```python
from build123d import *

# Parameters (mm, degrees)
BOSS_EXTRUDE1_DEPTH = 60.96
SKETCH2_R           = 3.302
BOSS_EXTRUDE2_DEPTH = 0.635


with BuildPart() as part:
    # Sketch1 → Boss-Extrude1 (new body)
    with BuildSketch(Plane.XY):
        with BuildLine():
            Line((0, 0.762), (3.048, 0.762))
            ThreePointArc((3.048, 0.762), (3.81, 0), (3.048, -0.762))
            Line((3.048, -0.762), (0, -0.762))
            ThreePointArc((0, -0.762), (-0.762, 0), (0, 0.762))
        make_face()
        with BuildLine():
            Line((2.286, 1.524), (2.286, -1.524))
            ThreePointArc((2.286, -1.524), (1.524, -2.286), (0.762, -1.524))
            Line((0.762, -1.524), (0.762, 1.524))
            ThreePointArc((0.762, 1.524), (1.524, 2.286), (2.286, 1.524))
        make_face()
    extrude(amount=BOSS_EXTRUDE1_DEPTH)

    # Sketch2 → Boss-Extrude2 (add)
    with BuildSketch(Plane(origin=(0, 0, 0), x_dir=(-1, 0, 0), z_dir=(0, 0, -1))):
        with Locations((-1.524, 0)):
            Circle(SKETCH2_R)
    extrude(amount=-BOSS_EXTRUDE2_DEPTH)


solid = part.part
```
Read the model definition and answer for the solid it produces. Units are mm, in the model's axes. A direction names the side the tool comes from. Give positions to 0.01 mm unless a question says otherwise; leave off trailing zeros. Loops run counter-clockwise (first coordinate to the right, second up) from the corner with the lowest first, then second, coordinate; pieces in that order, holes last.
Item 1: The part is cut by section A-A (y = 0). Write down the section's boundary in (x, z) (3 decimals).
Item 2: The part is cut by section B-B (z = 23.5). Write down the section's boundary in (x, y), and give its area (3 significant figures).
Item 3: Each of these flat-tipped pins is pushed along its axis until it touches: pin 1 Ø3 at (y, z) = (1, 32) entering from +X; pin 2 Ø0.8 at (y, z) = (1, 37) entering from -X; pin 3 Ø0.8 at (x, z) = (2.5, 35.5) entering from -Y. Where does it stop, or does it pass through?
Item 4: For faces 1 (the cylindrical face through (3.81, 0.02, 30.38)), 2 (the cylindrical face through (1.541, -2.286, 30.375)), 3 (the flat face through (0, 1, 0.635)), 4 (the cylindrical face through (-0.76, -0.02, 30.38)), 5 (the cylindrical face through (1.507, 2.286, 30.375)), determine the directions among +Z, -Z, +X, -X, +Y, -Y from which every point of the face is accessible in a straight line to the end or side of a thin tool.
Item 5: Find the intervals of material crossed by line 1 along Z through (x, y) = (4.25, 1.25) (3 decimals); line 2 along Y through (x, z) = (2.5, 49); line 3 along X through (y, z) = (1, 42), in increasing order.
Taken from the geometry:
1. outline: (-1.778, 0) - (4.826, 0) - (4.826, 0.635) - (3.81, 0.635) - (3.81, 60.96) - (-0.762, 60.96) - (-0.762, 0.635) - (-1.778, 0.635) - close
2. outline: (0, -0.76) - (0.76, -0.76) - (0.76, -1.52) arc R0.76 ccw to (2.29, -1.52) - (2.29, -0.76) - (3.05, -0.76) arc R0.76 ccw to (3.05, 0.76) - (2.29, 0.76) - (2.29, 1.52) arc R0.76 ccw to (0.76, 1.52) - (0.76, 0.76) - (0, 0.76) arc R0.76 ccw to start
2. area: 10.6 mm2
3. pin 1: stops at x = 3.81
3. pin 2: stops at x = -0.47
3. pin 3: stops at y = -2.02
4. face 1: +Z, +X
4. face 2: +Z, -Y
4. face 3: +Z
4. face 4: +Z, -X
4. face 5: +Z, +Y
5. line 1: z = 0 to 0.635
5. line 2: y = -0.76 to 0.76
5. line 3: x = 0.76 to 2.29
